Verification items for the finished model (mm, model axes). Face numbers are marked on the shaded views. A direction names the side the tool comes from. Coordinates: 2 decimals unless noted, no trailing zeros. Order: outer loops, then holes, each group sorted by start corner. A loop starts at its lowest first (then second) coordinate and runs counter-clockwise, first axis right, second up. Notation, with made-up numbers: (72.5, 86.5) -> (95.5, 86.5) arc R21 cw to (95.5, 100.5) -> close; hole circle Ø7 at (86, -5.75). An arc over 180 degrees is marked (long way). Use CSV: the item, a comma, the result in double quotes. Start each with the question number.
1) Sectioned sample at A-A on z = -5.5. Record the boundary of the cut face in (x, y), then the cut area to 3 significant figures.
2) Tool access check on the marked faces 4, 5 and 6. Record the directions out of +Z, -Z, +X, -X, +Y, -Y that give a thin tool (end or side, any length) a straight path to the whole face; none if there is none.
3) Sectioned sample at B-B on y = -2. Record the boundary of the cut face in (x, z) (3 decimals), then the cut area to 3 significant figures.
4) Sectioned sample at D-D on z = -26. Record the boundary of the cut face in (x, y), then the cut area to 3 significant figures.
5) Sectioned sample at C-C on x = 15.75. Record the boundary of the cut face in (y, z).
6) Scan lines: line 1 along Z through (x, y) = (3.25, -1.25); line 2 along Z through (x, y) = (11, 0.4); line 3 along Y through (x, z) = (10, -59) (3 decimals). Record each from-to range of solid material in increasing order.
7) Go/stop test with flat-tipped pins: pin 1 (3 mm diameter, centred on x = 20.5, z = -35, fed in from +Y); pin 2 (3 mm diameter, centred on x = 10, z = -55, fed in from -Y); pin 3 (1 mm diameter, centred on y = 1, z = -47, fed in from -X); pin 4 (1.8 mm diameter, centred on x = 20.5, z = -56, fed in from -Y). Record where each tip stops, or that it passes through.
8) Release check for a two-part mould opening along Z. For the marked faces 1, 2 and 3 record: released by +Z, released by -Z, zero draft, split by the parting line, or undercut.
from build123d import *

# Parameters (mm, degrees)
SKETCH1_W                                        = 61
SKETCH1_H                                        = 6.1
BOSS_EXTRUDE1_DEPTH                              = 22.5
SKETCH2_OUTSIDE_W                                = 76.06
SKETCH2_OUTSIDE_H                                = 21.16
SKETCH2_OUTSIDE_W_2                              = 61
SKETCH2_OUTSIDE_H_2                              = 5.41284
CUT_EXTRUDE1_DEPTH                               = 6
CUT_EXTRUDE3_DEPTH                               = 23.5
SKETCH6_R                                        = 3.175
CUT_EXTRUDE4_DEPTH                               = 7.1
SKETCH7_R                                        = 1.5
CUT_EXTRUDE5_DEPTH                               = 7.1
M2_5X0_45_TAPPED_HOLE1_D                         = 2.05
M2_5X0_45_TAPPED_HOLE2_D                         = 2.05
M2_5X0_45_TAPPED_HOLE2_DEPTH                     = 7.3
M2_5X0_45_TAPPED_HOLE2_TIP                       = 0.615882135
CBORE_FOR_M3_PAN_HEAD_MACHINE_SCREW1_D           = 3.4
CBORE_FOR_M3_PAN_HEAD_MACHINE_SCREW1_CBORE_D     = 6.5
CBORE_FOR_M3_PAN_HEAD_MACHINE_SCREW1_CBORE_DEPTH = 2.2


with BuildPart() as part:
    # Sketch1 → Boss-Extrude1 (new body)
    with BuildSketch(Plane(origin=(0, 0, 0), x_dir=(0, 0, -1), z_dir=(1, 0, 0))):
        with Locations((30.5, 0)):
            Rectangle(SKETCH1_W, SKETCH1_H)
    extrude(amount=BOSS_EXTRUDE1_DEPTH)

    # Sketch2 outside → Cut-Extrude1 (cut)
    with BuildSketch(Plane(origin=(22.5, 0, 0), x_dir=(0, 0, -1), z_dir=(1, 0, 0))):
        with Locations((30.5, 0)):
            Rectangle(SKETCH2_OUTSIDE_W, SKETCH2_OUTSIDE_H)
        with Locations((30.5, 0)):
            Rectangle(SKETCH2_OUTSIDE_W_2, SKETCH2_OUTSIDE_H_2, mode=Mode.SUBTRACT)
    extrude(amount=-CUT_EXTRUDE1_DEPTH, mode=Mode.SUBTRACT)

    # Sketch5 → Cut-Extrude3 (cut, through all)
    with BuildSketch(Plane.ZY):
        with BuildLine():
            Line((-43.5866, -0.01898), (-43.5866, -3.05))
            Line((-43.5866, -3.05), (-48.6514, -3.05))
            Line((-48.6514, -3.05), (-48.6514, -0.01898))
            ThreePointArc((-48.6514, -0.01898), (-46.119, 2.51342), (-43.5866, -0.01898))
        make_face()
    extrude(amount=-CUT_EXTRUDE3_DEPTH, mode=Mode.SUBTRACT)

    # Sketch6 → Cut-Extrude4 (cut, through all)
    with BuildSketch(Plane(origin=(0, 3.05, 0), x_dir=(1, 0, 0), z_dir=(0, 1, 0))):
        with Locations(Location((7.5, 30.5, 0), (0, 0, 270))):  # turned: the seam where the file's is
            Circle(SKETCH6_R)
    extrude(amount=-CUT_EXTRUDE4_DEPTH, mode=Mode.SUBTRACT)

    # Sketch7 → Cut-Extrude5 (cut, through all)
    with BuildSketch(Plane(origin=(0, 3.05, 0), x_dir=(1, 0, 0), z_dir=(0, 1, 0))):
        with Locations(Location((5, 55.5, 0), (0, 0, 270))):  # turned: the seam where the file's is
            Circle(SKETCH7_R)
        with Locations(Location((5, 5.5, 0), (0, 0, 270))):  # turned: the seam where the file's is
            Circle(SKETCH7_R)
    extrude(amount=-CUT_EXTRUDE5_DEPTH, mode=Mode.SUBTRACT)

    # M2.5x0.45 Tapped Hole1 (through all)
    with Locations(Plane(origin=(0, -3.05, 0), x_dir=(-1, 0, 0), z_dir=(0, -1, 0))):
        with Locations((-5, 18)):
            Hole(M2_5X0_45_TAPPED_HOLE1_D / 2)

    # M2.5x0.45 Tapped Hole2
    with Locations(Plane(origin=(0, 0, -61), x_dir=(-1, 0, 0), z_dir=(0, 0, -1))):
        with Locations((-10, 0)):
            Hole(M2_5X0_45_TAPPED_HOLE2_D / 2, depth=M2_5X0_45_TAPPED_HOLE2_DEPTH)
            with Locations((0, 0, -(M2_5X0_45_TAPPED_HOLE2_DEPTH + M2_5X0_45_TAPPED_HOLE2_TIP / 2))):  # 118° drill point
                Cone(0, M2_5X0_45_TAPPED_HOLE2_D / 2, M2_5X0_45_TAPPED_HOLE2_TIP, mode=Mode.SUBTRACT)

    # CBORE for M3 Pan Head Machine Screw1 (through all)
    with Locations(Plane(origin=(0, -3.05, 0), x_dir=(-1, 0, 0), z_dir=(0, -1, 0))):
        with Locations((-11, 55.228), (-11, 17.553)):
            CounterBoreHole(CBORE_FOR_M3_PAN_HEAD_MACHINE_SCREW1_D / 2, CBORE_FOR_M3_PAN_HEAD_MACHINE_SCREW1_CBORE_D / 2, CBORE_FOR_M3_PAN_HEAD_MACHINE_SCREW1_CBORE_DEPTH)


solid = part.part
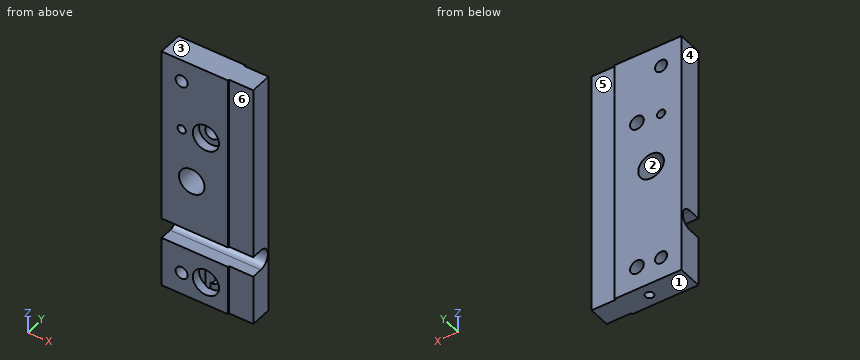
Answers follow:
1,outline,"(0, -3.05) -> (3.5, -3.05) -> (3.5, 3.05) -> (0, 3.05) -> close; (6.5, -3.05) -> (16.5, -3.05) -> (16.5, -2.71) -> (22.5, -2.71) -> (22.5, 2.71) -> (16.5, 2.71) -> (16.5, 3.05) -> (6.5, 3.05) -> close"
1,area,"115 mm²"
2,face 4,"+Z, -Z, -X, +Y, -Y"
2,face 5,"+Z, -Z, +X, +Y"
2,face 6,"+Z, -Z, +X, -Y"
3,outline,"(0, -61) -> (22.5, -61) -> (22.5, -48.651) -> (0, -48.651) -> close; (0, -43.587) -> (22.5, -43.587) -> (22.5, 0) -> (0, 0) -> close; hole circle Ø3 at (5, -55.5); hole circle Ø3 at (5, -5.5); hole circle Ø2.05 at (5, -18); hole circle Ø6.35 at (7.5, -30.5); hole circle Ø6.5 at (11, -55.228); hole circle Ø6.5 at (11, -17.553)"
3,area,"1,140 mm²"
4,outline,"(0, -3.05) -> (16.5, -3.05) -> (16.5, -2.71) -> (22.5, -2.71) -> (22.5, 2.71) -> (16.5, 2.71) -> (16.5, 3.05) -> (0, 3.05) -> close"
4,area,"133 mm²"
5,outline,"(-3.05, -61) -> (3.05, -61) -> (3.05, 0) -> (-3.05, 0) -> (-3.05, -43.59) -> (-0.02, -43.59) arc R2.53 cw to (-0.02, -48.65) -> (-3.05, -48.65) -> close"
6,line 1,"z = -61 to -48.65, -43.59 to 0"
6,line 2,"z = -61 to -56.93, -53.53 to -48.62, -43.62 to -19.25, -15.85 to 0"
6,line 3,"y = -3.05 to -1.025, 1.025 to 3.05"
7,pin 1,"stops at y = 2.71"
7,pin 2,"stops at y = -0.85"
7,pin 3,"passes through"
7,pin 4,"stops at y = -2.71"
8,face 1,"released by -Z"
8,face 2,"undercut"
8,face 3,"released by +Z"
